Source: CAD feature listing. Evaluate the final solid. Frame: model axes, mm. Give positions to 0.01 mm unless a question says otherwise; leave off trailing zeros. Order: outer loops, then holes, each group sorted by start corner. A loop starts at its lowest first (then second) coordinate and runs counter-clockwise, first axis right, second up. Notation, with made-up numbers: M 86,-21 L 104,-21 A23 ccw 104,5 Z; hole C 29,49 d4. An arc over 180 degrees is marked long. Use CSV: the item, a comma, the result in double quotes. Start each with the question number.
1. Line query: line 1 along Y through (x, z) = (89, 1.55); line 2 along Z through (x, y) = (-21, -0.5); line 3 along Z through (x, y) = (-47, 16.5). Output: solid intervals per line, ascending. Write a range as [from, to].
2. Section query B-B, the plane y = -6. Return the cut outline in (x, z), plus the area to 3 significant figures.
3. Section query A-A, the plane x = -20. Return the cut outline in (y, z).
4. Pin query (flat end, axial travel): P1, Ø8, axis at x = -74, y = 10, coming from the +Z side. Return the tip coordinate at first contact, or that it passes through.
5. Mould query, pull axis Y, two halves, no side actions, for faces 1 (the flat face through (-2, 0, 0)), 2 (the flat face through (-2, 0, 1)). Classes: released by +Y, released by -Y, zero draft, split by the parting line, or undercut.
from build123d import *

# Parameters (mm, degrees)
F0_W     = 230
F0_H     = 38
F1_DEPTH = 1
F2_W     = 230
F2_H     = 1.25
F3_DEPTH = 0.5
F4_W     = 230
F4_H     = 3
F5_DEPTH = 0.5


with BuildPart() as f1:
    # F0 (on Top) → F1 (new body)
    with BuildSketch(Plane.XY):
        Rectangle(F0_W, F0_H)
    extrude(amount=F1_DEPTH)

    # F2 (on face) → F3 (join)
    with BuildSketch(Plane.XY.offset(1)):
        with Locations((0, 18.375)):
            Rectangle(F2_W, F2_H)
        with Locations((0, -18.375)):
            Rectangle(F2_W, F2_H)
    extrude(amount=F3_DEPTH)

    # F4 (on face) → F5 (join)
    with BuildSketch(Plane.XY.offset(1.5)):
        with Locations((0, 17.5)):
            Rectangle(F4_W, F4_H)
        with Locations((0, -17.5)):
            Rectangle(F4_W, F4_H)
    extrude(amount=F5_DEPTH)


solid = f1.part
Result set:
1,line 1,"[-19, -16], [16, 19]"
1,line 2,"[0, 1]"
1,line 3,"[0, 1], [1.5, 2]"
2,outline,"M -115,0 L 115,0 L 115,1 L -115,1 Z"
2,area,"230 mm2"
3,outline,"M -19,0 L 19,0 L 19,2 L 16,2 L 16,1.5 L 17.75,1.5 L 17.75,1 L -17.75,1 L -17.75,1.5 L -16,1.5 L -16,2 L -19,2 Z"
4,P1,"z = 1"
5,face 1,"zero draft"
5,face 2,"undercut"
